Could you check a few things on this drawing? It's one solid part, dimensions in mm from its lowest x, y, z. Round coordinates to 2 decimals unless told otherwise and drop trailing zeros. Order: outer loops, then holes, each group sorted by start corner. A loop starts at its lowest first (then second) coordinate and runs counter-clockwise, first axis right, second up.
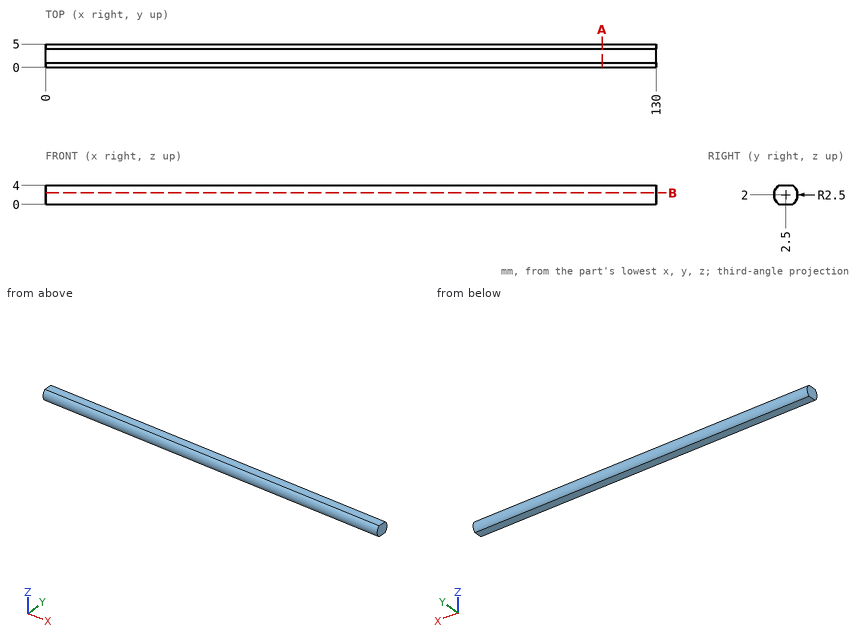
1) I need wall thicknesses on line 1 (Y direction, x = 15, z = 2.1); line 2 (Y direction, x = 66, z = 3.1) (3 decimals); line 3 (Z direction, x = 74.5, y = 4.5). Which ranges of each line are inside material? Lowest first, please.
2) If we section it at B-B (z = 2.45): Write out the boundary of the cut face in (x, y).
3) If we section it at A-A (x = 118.5): Write out the boundary of the cut face in (y, z), plus the area to 3 significant figures.
Solutions:
1. line 1: y = 0 to 5
1. line 2: y = 0.255 to 4.745
1. line 3: z = 0.5 to 3.5
2. outline: (0, 0.04) - (130, 0.04) - (130, 4.96) - (0, 4.96) - close
3. outline: (1, 0) - (4, 0) arc R2.5 ccw to (4, 4) - (1, 4) arc R2.5 ccw to start
3. area: 17.6 mm2
